Here's how the part is built. I have some questions about the finished solid (model axes, mm). A direction names the side the tool comes from. Round coordinates to 2 decimals unless told otherwise and drop trailing zeros. Loops run counter-clockwise (first coordinate to the right, second up) from the corner with the lowest first, then second, coordinate; pieces in that order, holes last. Notation, with made-up numbers: M 16.5,82 L 73.5,82 A21 cw 73.5,102 Z; hole C 69.5,38 d4. An arc over 180 degrees is marked long. Answer as CSV lines item,"result".
```python
from build123d import *

# Parameters (mm, degrees)
F0_R          = 3.15
F0_R_2        = 3.65
F1_DEPTH      = 25
F2_R          = 3.1
F3_DEPTH      = 17.301
F3_DEPTH_BACK = 40.501
F2_R_2        = 4.25
F4_DEPTH      = 0.5
F5_R          = 4.25
F5_R_2        = 3.1
F6_DEPTH      = 0.5
F7_W          = 20.65
F7_H          = 20
F8_DEPTH      = 22.3
F9_W          = 20.65
F9_H          = 20
F10_DEPTH     = 12.3
F11_R         = 2.65
F12_DEPTH     = 25.001
F13_T         = 2.5
F13_T3_DEPTH  = 27.3
F13_T5_DEPTH  = 25.65
F13_T7_DEPTH  = 30
F13_T9_DEPTH  = 25
F13_T11_DEPTH = 17.3


# Not quite as in the source:
# - a shell that OpenCascade refuses in one call is made with other operations: the cavity is built on its own and cut out


with BuildPart() as f1:
    # F0 (on Front) → F1 (new body)
    with BuildSketch(Plane.XZ):
        Polygon((4.35, 29.15), (-8.65, 29.15), (-8.65, -28.65), (4.35, -28.65), (25, -16.35), (25, -11.35), (1, -11.35), (1, 1.85), (25, 1.85), (25, 6.85), align=None)
        with Locations((0, -22.5)):
            Circle(F0_R, mode=Mode.SUBTRACT)
        with Locations((0, 22.5)):
            Circle(F0_R_2, mode=Mode.SUBTRACT)
    extrude(amount=F1_DEPTH)

    # F2 (on face) → F3 (cut, two sides)
    with BuildSketch(Plane.XY.offset(-11.35)) as f3_sk:
        with Locations((13, -13)):
            Circle(F2_R)
    extrude(amount=-F3_DEPTH, mode=Mode.SUBTRACT)
    extrude(f3_sk.sketch, amount=F3_DEPTH_BACK, mode=Mode.SUBTRACT)

    # F2 (on face) → F4 (join)
    with BuildSketch(Plane.XY.offset(-11.35)):
        with Locations((13, -13)):
            Circle(F2_R_2)
        with Locations((13, -13)):
            Circle(F2_R, mode=Mode.SUBTRACT)
    extrude(amount=F4_DEPTH)

    # F5 (on face) → F6 (join)
    with BuildSketch(Plane(origin=(0, 0, 1.85), x_dir=(1, 0, 0), z_dir=(0, 0, -1))):
        with Locations((13, 13)):
            Circle(F5_R)
        with Locations((13, 13)):
            Circle(F5_R_2, mode=Mode.SUBTRACT)
    extrude(amount=F6_DEPTH)

    # F7 (on face) → F8 (cut)
    with BuildSketch(Plane.XY.offset(29.15)):
        with Locations((14.675, -12.5)):
            Rectangle(F7_W, F7_H)
    extrude(amount=-F8_DEPTH, mode=Mode.SUBTRACT)

    # F9 (on face) → F10 (cut)
    with BuildSketch(Plane(origin=(0, 0, -28.65), x_dir=(1, 0, 0), z_dir=(0, 0, -1))):
        with Locations((14.675, 12.5)):
            Rectangle(F9_W, F9_H)
    extrude(amount=-F10_DEPTH, mode=Mode.SUBTRACT)

    # F11 (on face) → F12 (cut, through all)
    with BuildSketch(Plane.XZ.offset(25)):
        with Locations((-3.85, -4.75)):
            Circle(F11_R)
    extrude(amount=-F12_DEPTH, mode=Mode.SUBTRACT)

    # F13: shell of thickness 2.5, made by hand


with BuildPart() as f13_core1:
    # F13_t2: copy of F1
    add(f1.part)

    # the walls: a layer under each face that stays
    f13_faces = [f13_core1.faces().sort_by_distance(p)[0] for p in [
        (14.675, -1.25, 18),
        (-3.0416666667, 0, -19.0166666667),
        (-2.15, -12.5, 29.15),
        (14.675, -2.5, 10.5666666667),
        (25, -12.5, 4.35),
        (5, -20.8333333333, 1.85),
        (1, -12.5, -4.75),
        (-2.15, -12.5, -28.65),
        (21, -20.8333333333, -11.35),
        (14.675, -1.25, -22.5),
        (25, -12.5, -13.85),
        (-6.5, -12.5, -4.75),
        (-3.15, -12.5, -22.5),
        (-3.65, -12.5, 22.5),
        (4.35, -12.5, 18),
        (14.675, -23.75, 18),
        (-3.0416666667, -25, -19.0166666667),
        (7.7916666667, -19.1666666667, 6.85),
        (8.75, -13, 1.6),
        (4.35, -12.5, -22.5),
        (14.675, -23.75, -22.5),
        (8.75, -13, -11.1),
        (7.7916666667, -2.5, -18.4),
        (7.7916666667, -5.8333333333, -16.35),
        (7.7916666667, -22.5, 10.5666666667),
        (9.9, -13, 4.35),
        (10.1666666667, -10.1666666667, 1.35),
        (14.675, -22.5, -18.4),
        (10.1666666667, -15.8333333333, -10.85),
        (9.9, -13, -13.85),
        (9.9, -13, 1.6),
        (9.9, -13, -11.1),
    ]]
    thicken(f13_faces, amount=-F13_T, mode=Mode.SUBTRACT)

    # F13_s4 → F13_t3 (cut)
    with BuildSketch(Plane.XY.offset(4.35)):
        Polygon((4.375, -2.525), (4.35, 0), (1.85, 0), (1.85, -2.5), align=None)
        Polygon((4.375, -22.475), (1.85, -22.5), (1.85, -25), (4.35, -25), align=None)
    extrude(amount=F13_T3_DEPTH, mode=Mode.SUBTRACT)

    # F13_s6 → F13_t5 (cut)
    with BuildSketch(Plane.YZ.offset(1.85)):
        Polygon((-2.525, 6.875), (0, 6.85), (0, 4.35), (-2.5, 4.35), align=None)
        Polygon((-22.475, 6.875), (-22.5, 4.35), (-25, 4.35), (-25, 6.85), align=None)
        Polygon((-2.525, -16.375), (0, -16.35), (0, -13.85), (-2.5, -13.85), align=None)
        Polygon((-22.475, -16.375), (-22.5, -13.85), (-25, -13.85), (-25, -16.35), align=None)
    extrude(amount=F13_T5_DEPTH, mode=Mode.SUBTRACT)

    # F13_s8 → F13_t7 (cut)
    with BuildSketch(Plane.XZ.offset(-2.5)):
        Polygon((1.025, 1.825), (1, 4.35), (-1.5, 4.35), (-1.5, 1.85), align=None)
        Polygon((1.025, -11.325), (-1.5, -11.35), (-1.5, -13.85), (1, -13.85), align=None)
    extrude(amount=F13_T7_DEPTH, mode=Mode.SUBTRACT)

    # F13_s10 → F13_t9 (cut)
    with BuildSketch(Plane.XZ):
        Polygon((4.375, 6.875), (1.85, 6.85), (1.85, 4.35), (4.35, 4.35), align=None)
        Polygon((4.375, -16.375), (1.85, -16.35), (1.85, -13.85), (4.35, -13.85), align=None)
    extrude(amount=F13_T9_DEPTH, mode=Mode.SUBTRACT)

    # F13_s12 → F13_t11 (cut)
    with BuildSketch(Plane.XY.offset(-31.15)):
        Polygon((4.375, -22.475), (1.85, -22.5), (1.85, -25), (4.35, -25), align=None)
        Polygon((4.375, -2.525), (1.85, -2.5), (1.85, 0), (4.35, 0), align=None)
    extrude(amount=F13_T11_DEPTH, mode=Mode.SUBTRACT)

    # F13_s13 → F13_t14 (revolve, cut)
    with BuildSketch(Plane.XZ.offset(13)):
        Polygon((17.275, 1.825), (17.25, 4.35), (14.75, 4.35), (14.75, 1.85), align=None)
    revolve(axis=Axis((13, -13, 1.85), (0, 0, -1)), mode=Mode.SUBTRACT)

    # F13_s15 → F13_t16 (revolve, cut)
    with BuildSketch(Plane.XZ.offset(13)):
        Polygon((17.275, -11.325), (17.25, -13.85), (14.75, -13.85), (14.75, -11.35), align=None)
    revolve(axis=Axis((13, -13, -11.35), (0, 0, 1)), mode=Mode.SUBTRACT)


with BuildPart() as f1_1:
    add(f1.part)

    # what is left inside the walls is the cavity
    f13_cavity = [f13_core1.part.solids().sort_by_distance(p)[0] for p in [
        (-8.625, -15.833333, 11.883073),
        (-8.625, -15.833333, -16.383073),
    ]]
    add(f13_cavity, mode=Mode.SUBTRACT)


solid = f1_1.part
```
1. We'd pull the mould along Z, two halves only. Please class faces 4 (the flat face through (10.2, -9.5, 1.85)), 5 (the flat face through (14.82, -1.232, 17.844)), 6 (the flat face through (10, -2.5, 13)): pulls with the +Z half, pulls with the -Z half, needs draft (parallel to the pull), parting line crosses it, or undercut.
Evaluation:
face 4,"undercut"
face 5,"pulls with the +Z half"
face 6,"needs draft"
2. If I drill on line 1 (Z direction, x = 0, y = -19.5); line 2 (Z direction, x = 12, y = -21.5); line 3 (Y direction, x = 13, z = 3.45), over which ranges is the centre line in solid material (lowest first)? Write a range as [from, to].
Evaluation:
line 1,"z = [-28.65, -25.65], [-19.35, -16.85], [-13.85, 4.35], [16.35, 18.85], [26.15, 29.15]"
line 2,"z = [-16.35, -11.35], [1.85, 6.85]"
line 3,"y = [-25, -16.1], [-9.9, 0]"
3. I want a section at A-A, the plane z = 22.5. Please give me the cut outline in (x, y).
Evaluation:
outline,"M -8.65,-25 L -3.65,-25 L -3.65,0 L -8.65,0 L -8.65,-2.5 L -6.15,-2.5 L -6.15,-22.5 L -8.65,-22.5 Z; M 3.65,-25 L 10.51,-25 L 10.51,-22.5 L 4.35,-22.5 L 4.35,-2.5 L 10.51,-2.5 L 10.51,0 L 3.65,0 Z"
4. I want a section at C-C, the plane y = -5.5. Count the separate pieces of the cut face and the enclosed holes in it, and give its area (3 significant figures).
Evaluation:
separate pieces,"1"
enclosed holes,"3"
area,"522 mm²"
5. I want a section at D-D, the plane z = -13. Please give me the cut outline in (x, y).
Evaluation:
outline,"M -8.65,-25 L 25,-25 L 25,0 L -8.65,0 L -8.65,-2.5 L -1.5,-2.5 L -1.5,-22.5 L -8.65,-22.5 Z; hole C 13,-13 d6.2"
6. For P1, Ø1, axis at y = -17, z = -16, coming from the -X side; P2, Ø12, axis at y = -7, z = 13, coming from the +X side; P3, Ø4, axis at x = 9, y = -13.5, coming from the -Z side, each with a flat end and sliding along its axis, tell me the tip position at first contact or that it passes through.
Evaluation:
P1,"stops at x = 1.85"
P2,"stops at x = 22.98"
P3,"stops at z = -16.35"
7. Which directions (+Z, -Z, +X, -X, +Y, -Y) give clear straight access to the entire face, cutting with the end or side of a thin tool? Please do faces 1 (the flat face through (-7, -12, 26.65)), 2 (the cylindrical face through (-5.74, -12.64, -9.54)), 3 (the flat face through (10, -22.5, -20)).
Evaluation:
face 1,"-X"
face 2,"none"
face 3,"-Z, +X"
8. I want a section at B-B, the plane x = 7.5. Please give me the cut outline in (y, z).
Evaluation:
outline,"M -25,-26.77 L -22.5,-26.77 L -22.5,-16.35 L -2.5,-16.35 L -2.5,-26.77 L 0,-26.77 L 0,-11.35 L -25,-11.35 Z; M -25,1.85 L 0,1.85 L 0,25.75 L -2.5,25.75 L -2.5,6.85 L -22.5,6.85 L -22.5,25.75 L -25,25.75 Z"
